Read the model definition and answer for the solid it produces. Units are mm, in the model's axes. Face numbers are marked on the shaded views. A direction names the side the tool comes from. Coordinates: 2 decimals unless noted, no trailing zeros. Loops run counter-clockwise (first coordinate to the right, second up) from the corner with the lowest first, then second, coordinate; pieces in that order, holes last. Notation, with made-up numbers: M 38.25,13 L 82.25,13 A18 cw 82.25,30 Z; hole C -23.5,-34 d4. An arc over 180 degrees is marked long. Put each result on its own line as item: value.
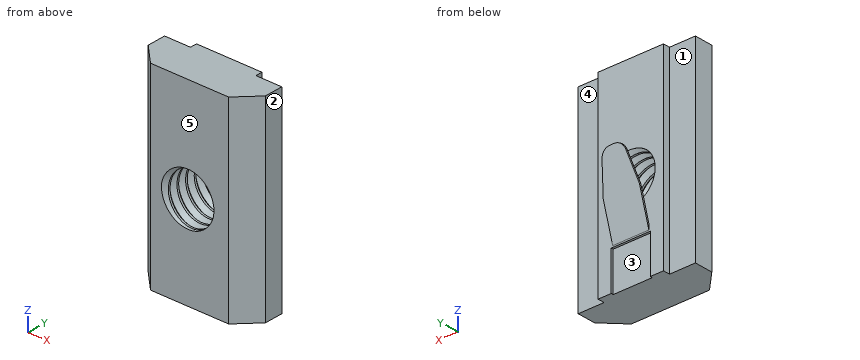
from build123d import *

# Parameters (mm, degrees)
EXTRUDE_1_DEPTH      = 20
CHAMFER_1_SIZE       = 2
SKETCH_2_R           = 2.5
CUT_EXTRUDE_1_DEPTH  = 22.381300241
SWEEP_1_PITCH        = 1
SKETCH_6_W           = 4
SKETCH_6_H           = 0.46098281
CUT_EXTRUDE_2_DEPTH  = 4
EXTRUDE_2_DEPTH      = 1.85
EXTRUDE_2_DEPTH_BACK = 1.85
CUT_EXTRUDE_3_DEPTH  = 1.85
FILLET_1_R           = 1


with BuildPart() as part:
    # 草图1 → 凸台-拉伸1 (new body)
    with BuildSketch(Plane.XY):
        Polygon((-6, 0), (6, 0), (6, 3.9), (3.35, 3.9), (3.35, 4.6), (-3.35, 4.6), (-3.35, 3.9), (-6, 3.9), align=None)
    extrude(amount=EXTRUDE_1_DEPTH)

    # 倒角1
    chamfer_1_edges = [part.edges().sort_by_distance(p)[0] for p in [
        (6, 0, 10),
        (-6, 0, 10),
    ]]
    chamfer(chamfer_1_edges, length=CHAMFER_1_SIZE)

    # 草图2 → 切除-拉伸1 (cut, through all)
    with BuildSketch(Plane(origin=(0, 4.6, 0), x_dir=(1, 0, 0), z_dir=(0, 1, 0))):
        with Locations(Location((0, -9.419001614, 0), (0, 0, 270))):
            Circle(SKETCH_2_R)
    extrude(amount=-CUT_EXTRUDE_1_DEPTH, mode=Mode.SUBTRACT)

    # 切除-扫描1: arcs per turn and ends read off the stored shape
    # 切除-扫描1: the profile of 草图5 profile screwed along a right-hand helix through 5 turns, 8 arcs to a turn; built about Z, then put on its axis
    sweep_1_z = Axis((0, 0, 0), (0, 0, 1))
    sweep_1_corners = [(2.4997, 0, -0.4003), (2.4997, 0, 0.4003), (2.9, 0, 0)]
    with BuildLine(mode=Mode.PRIVATE) as sweep_1_profile:
        Line(sweep_1_corners[0], sweep_1_corners[1])
        Line(sweep_1_corners[1], sweep_1_corners[2])
        Line(sweep_1_corners[2], sweep_1_corners[0])
    sweep_1_cap = Face(sweep_1_profile.wire())
    sweep_1_turn_angles = [0, 22.5, 45, 67.5, 90, 112.5, 135, 157.5, 180, 202.5, 225, 247.5, 270, 292.5, 315, 337.5, 360]
    sweep_1_turn_weights = [1, 0.9238795325112867, 1, 0.9238795325112867, 1, 0.9238795325112867, 1, 0.9238795325112867, 1, 0.9238795325112867, 1, 0.9238795325112867, 1, 0.9238795325112867, 1, 0.9238795325112867, 1]
    sweep_1_turn_rails = [Edge.make_bspline([Vector(p[0], p[1], 0).rotate(sweep_1_z, sweep_1_turn_angles[k]) / sweep_1_turn_weights[k] + Vector(0, 0, p[2] + SWEEP_1_PITCH * sweep_1_turn_angles[k] / 360) for k in range(17)], [0, 0, 0, 1, 1, 2, 2, 3, 3, 4, 4, 5, 5, 6, 6, 7, 7, 8, 8, 8], 2, sweep_1_turn_weights) for p in sweep_1_corners]
    sweep_1_turn_sides = [Face.make_surface_from_curves(sweep_1_turn_rails[p[0]], sweep_1_turn_rails[p[1]]) for p in [(0, 1), (1, 2), (2, 0)]]
    sweep_1 = Plane(origin=(0, 4.6, 9.419001614), x_dir=(0.7071067811865438, 0, -0.7071067811865513), z_dir=(0, -1, 0)) * Solid(Shell([*[p.moved(Location((0, 0, SWEEP_1_PITCH * i))) for i in range(5) for p in sweep_1_turn_sides], sweep_1_cap, sweep_1_cap.rotate(sweep_1_z, 1800).moved(Location((0, 0, SWEEP_1_PITCH * 1800 / 360)))]))
    add(sweep_1, mode=Mode.SUBTRACT)

    # 草图6 → 切除-拉伸2 (cut)
    with BuildSketch(Plane(origin=(0, 0, 0), x_dir=(-1, 0, 0), z_dir=(0, 0, -1))):
        with Locations((0, 4.6)):
            Rectangle(SKETCH_6_W, SKETCH_6_H)
    extrude(amount=-CUT_EXTRUDE_2_DEPTH, mode=Mode.SUBTRACT)

    # 草图7 → 凸台-拉伸2 (add, two sides: drawn at the far end of the back side and taken through both)
    with BuildSketch(Plane(origin=(0, 0, 0), x_dir=(0, 0, -1), z_dir=(1, 0, 0)).offset(-EXTRUDE_2_DEPTH_BACK)):
        Polygon((-4.154281608, 4.6), (-11.466055335, 6.795870295), (-11.514546749, 6.63440436), (-4.740419706, 4.6), align=None)
    extrude(amount=EXTRUDE_2_DEPTH + EXTRUDE_2_DEPTH_BACK)

    # 草图8 → 切除-拉伸3 (cut)
    with BuildSketch(Plane(origin=(0, 3.075042872, -0.923496206), x_dir=(1, 0, 0), z_dir=(0, 0.9577419497796025, -0.2876288539635158))):
        Polygon((-1.85, -9.119016537), (-1.041199164, -12.936210577), (-1.85, -12.936210577), align=None)
    cut_extrude_3 = extrude(amount=-CUT_EXTRUDE_3_DEPTH, mode=Mode.SUBTRACT)

    # 镜向1: 切除-拉伸3 across plane
    add(cut_extrude_3.mirror(Plane(origin=(0, 0, 0), x_dir=(0, 0, 1), z_dir=(1, 0, 0))), mode=Mode.SUBTRACT)

    # 圆角1
    fillet_1_edges = [part.edges().sort_by_distance(p)[0] for p in [
        (-1.041199164, 6.715137327, 11.490301042),
        (1.041199164, 6.715137327, 11.490301042),
    ]]
    fillet(fillet_1_edges, radius=FILLET_1_R)


solid = part.part
1) Straight lines are drawn through the part: line 1 (Y direction, x = -2.5, z = 10.5); line 2 (X direction, y = 1.75, z = 11.5); line 3 (Y direction, x = 3, z = 12). For each, find the intervals that lie inside material, in ascending order. Write a range as [from, to].
Answer list:
line 1: y = [0.22, 0.86], [1.22, 1.86], [2.22, 2.86], [3.22, 3.86], [4.22, 4.6]
line 2: x = [-5.75, -1.42], [1.39, 5.75]
line 3: y = [0, 4.6]
2) Find section B-B, the plane z = 8.5. Count the separate pieces of the cut face and the enclosed holes in it, plus the area to 3 significant figures.
Answer list:
separate pieces: 3
enclosed holes: 0
area: 25.2 mm^2
3) Which of the six approach directions +Z, -Z, +X, -X, +Y, -Y give full straight-line access (tool end or side, diameter ignored) to the marked faces 4 and 5?
Answer list:
face 4: +Z, -Z, +X, +Y
face 5: +Z, -Z, +X, -X, -Y
4) Determine the mould class of the marked faces 1, 2 and 3 for opening direction X: released by +X, released by -X, zero draft, split by the parting line, or undercut.
Answer list:
face 1: zero draft
face 2: released by +X
face 3: undercut
5) Given pin 1 Ø3 at (y, z) = (5, 18) entering from +X; pin 2 Ø3 at (x, z) = (-4.5, 6.5) entering from +Y; pin 3 Ø2 at (y, z) = (5.5, 17) entering from -X; pin 4 Ø2 at (x, z) = (-1.5, 9) entering from -Y, each flat-ended and moving along its own axis, determine where each tip first touches the part or whether it passes through.
Answer list:
pin 1: stops at x = 6
pin 2: stops at y = 4.6
pin 3: stops at x = -3.35
pin 4: stops at y = 0.27
6) Find section A-A, the plane z = 3. Write down the section's boundary in (x, y), plus the area to 3 significant figures.
Answer list:
outline: M -6,2 L -4,0 L 4,0 L 6,2 L 6,3.9 L 3.35,3.9 L 3.35,4.6 L 2,4.6 L 2,4.37 L -2,4.37 L -2,4.6 L -3.35,4.6 L -3.35,3.9 L -6,3.9 Z
area: 46.6 mm^2
7) Find section C-C, the plane y = 6. Write down the section's boundary in (x, z).
Answer list:
outline: M -1.63,8.82 L 1.63,8.82 L 1.51,9.4 L -1.51,9.4 Z
